Here's the drawing with two shaded views (mm, measured from the low corner). I have some questions. A direction names the side the tool comes from. Coordinates: 2 decimals unless noted, no trailing zeros. Write each loop counter-clockwise with the first axis right and the second up, starting at its lowest first coordinate (ties: lowest second). Pieces come first, ordered by that corner, then holes.
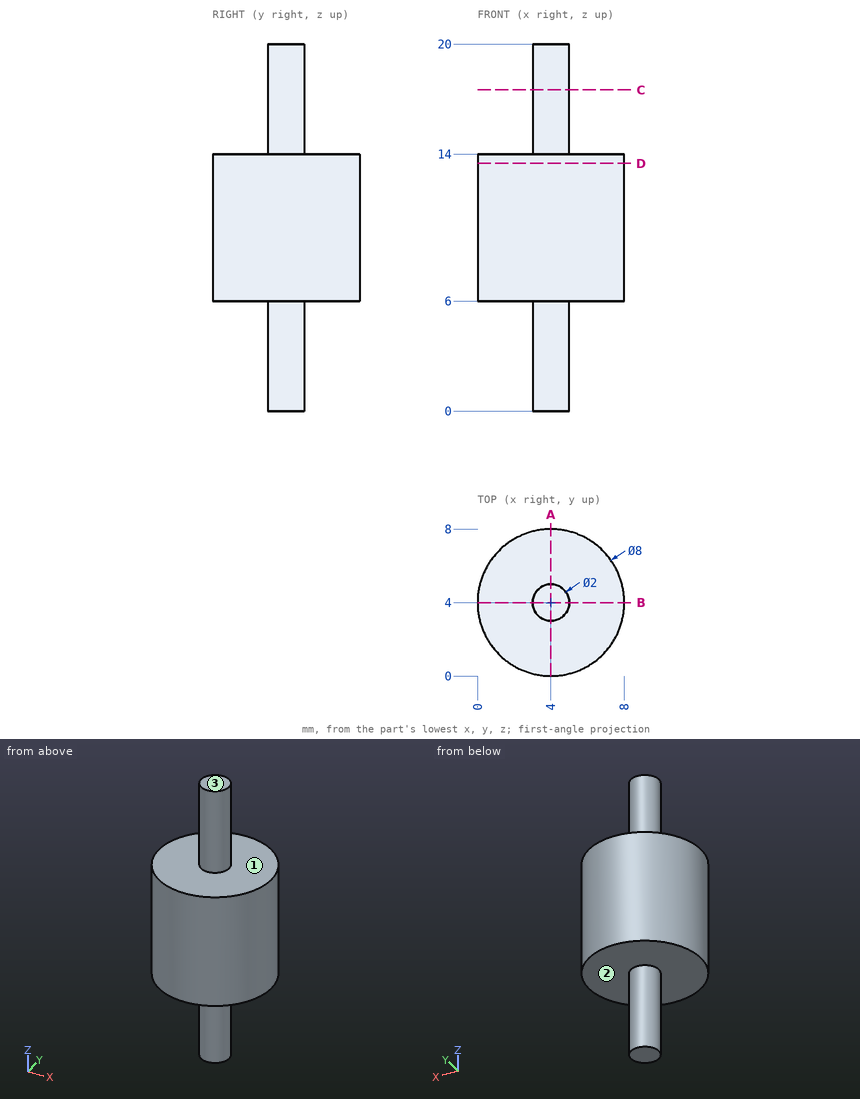
1. On a 3-axis mill with a long thin cutter (end or side, diameter ignored), from which of +Z, -Z, +X, -X, +Y, -Y can I reach the whole of each face in a straight line? I mean the marked faces 1, 2 and 3. Say none if no direction works.
Verdict:
face 1: +Z
face 2: -Z
face 3: +Z, +X, -X, +Y, -Y
2. I want a section at A-A on x = 4. Please give me the cut outline in (y, z), plus the area to 3 significant figures.
Verdict:
outline: (0, 6) - (3, 6) - (3, 0) - (5, 0) - (5, 6) - (8, 6) - (8, 14) - (5, 14) - (5, 20) - (3, 20) - (3, 14) - (0, 14) - close
area: 88.0 mm2
3. I want a section at C-C on z = 17.5. Please give me the cut outline in (x, y).
Verdict:
outline: circle Ø2 at (4, 4)
4. I want a section at D-D on z = 13.5. Please give me the cut outline in (x, y), plus the area to 3 significant figures.
Verdict:
outline: circle Ø8 at (4, 4)
area: 50.3 mm2
5. Please list where these lines run through material, in increasing order: line 1 along Z through (x, y) = (4.25, 2.75); line 2 along Y through (x, z) = (3, 8); line 3 along X through (y, z) = (6.25, 8.5).
Verdict:
line 1: z = 6 to 14
line 2: y = 0.13 to 7.87
line 3: x = 0.69 to 7.31
6. For pin 1 (1.5 mm diameter, centred on x = 3.5, y = 6.5, fed in from +Z), with a flat end and sliding along its axis, tell me the tip position at first contact or that it passes through.
Verdict:
pin 1: stops at z = 14
